The model under review builds one solid part; all positions refer to its coordinate system, in mm. Face numbers are marked on the shaded views. A direction names the side the tool comes from. Coordinates: 2 decimals unless noted, no trailing zeros. Write each loop counter-clockwise with the first axis right and the second up, starting at its lowest first coordinate (ties: lowest second). Pieces come first, ordered by that corner, then holes. Notation, with made-up numbers: (11, -31) - (22, -31) arc R18 ccw to (22, -13) - close; hole circle Ø10 at (62, 86.5). An arc over 180 degrees is marked (long way). Return JSON: item names as keys, results as strings. Group by question number.
(1) We need section B-B on z = 4.25. State the section outline as (x, y) points.
(2) Draft analysis for pull direction Y (two halves, no side actions). For the marked faces 1, 2 and 3, state which applies: released by +Y, released by -Y, zero draft, split by the parting line, or undercut.
(3) Tool access review of the marked faces 4, 5, 6 and 7: name each direction out of +Z, -Z, +X, -X, +Y, -Y from which nothing blocks a thin tool from reaching the whole face with its end or side.
(4) For pin 1 Ø6.5 at (x, y) = (-31, -5) entering from +Z; pin 2 Ø4 at (x, y) = (-38.5, -3) entering from -Z; pin 3 Ø2 at (x, y) = (-10.5, 3.5) entering from +Z, all flat-tipped, find the tip position at first contact; note any pin that passes through.
(5) We need section A-A on x = 0. State the section outline as (y, z) points, then the cut area to 4 significant figures.
(6) We need section C-C on y = -14.75. State the section outline as (x, z) points, then the cut area to 3 significant figures.
(7) To check wall thickness, follow L1, parallel to Y at x = -14, z = 0.75; L2, parallel to Y at x = 2.5, z = 7.5; L3, parallel to Z at x = -11.5, y = 6.5. State the ranges of each line that lie inside material, in increasing order. Write a range as from..to.
(8) We need section D-D on x = -22.5. State the section outline as (y, z) points, then the cut area to 3 significant figures.
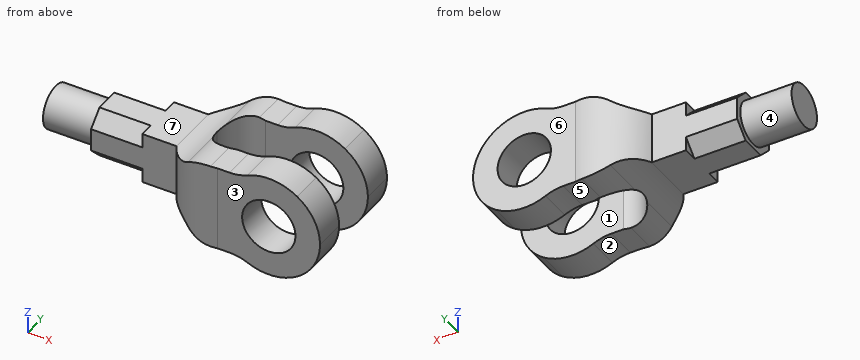
```python
from build123d import *

# Parameters (mm, degrees)
SKETCH4_R               = 12
SKETCH4_R_2             = 6.25
BOSS_EXTRUDE2_DEPTH     = 7.5
BOSS_EXTRUDE3_DEPTH     = 10
SKETCH6_R               = 6.25
CUT_EXTRUDE1_DEPTH      = 20
SKETCH7_W               = 20
SKETCH7_H               = 7.5
BOSS_EXTRUDE4_DEPTH     = 5.36675
CUT_EXTRUDE2_DEPTH      = 50.133277179
CUT_EXTRUDE2_DEPTH_BACK = 50.133277179
FILLET1_R               = 10
FILLET2_R               = 10
CUT_EXTRUDE3_DEPTH      = 12
SKETCH10_R              = 5
BOSS_EXTRUDE5_DEPTH     = 12
FILLET3_R               = 10


with BuildPart() as part:
    # Sketch4 → Boss-Extrude2 (new body)
    with BuildSketch(Plane(origin=(0, 0, 0), x_dir=(1, 0, 0), z_dir=(0, 1, 0))):
        with Locations(Location((0, 0, 0), (0, 0, 270))):
            Circle(SKETCH4_R)
        with Locations(Location((0, 0, 0), (0, 0, 270))):
            Circle(SKETCH4_R_2, mode=Mode.SUBTRACT)
    extrude(amount=BOSS_EXTRUDE2_DEPTH)

    # Sketch5 → Boss-Extrude3 (add, symmetric)
    with BuildSketch(Plane.XY):
        with BuildLine():
            Line((-25.749055866, 0.593145751), (-45.749055866, 0.593145751))
            Line((-45.749055866, 0.593145751), (-45.749055866, -5.656854249))
            Line((-45.749055866, -5.656854249), (-20, -5.656854249))
            ThreePointArc((-20, -5.656854249), (-17.464101615, -0.757874764), (-12, 0))
            Line((-12, 0), (12, 0))
            Line((12, 0), (12, 7.5))
            Line((12, 7.5), (-12, 7.5))
            ThreePointArc((-12, 7.5), (-19.973874913, 6.234976235), (-25.749055866, 0.593145751))
        make_face()
    extrude(amount=BOSS_EXTRUDE3_DEPTH, both=True)

    # Sketch6 → Cut-Extrude1 (cut)
    with BuildSketch(Plane.XZ):
        with BuildLine():
            Line((6.633249581, -10), (12, -10))
            Line((12, -10), (12, 0))
            ThreePointArc((12, 0), (10.573528147, -5.674548662), (6.633249581, -10))
        make_face()
        with BuildLine():
            ThreePointArc((6.633249581, 10), (10.573528147, 5.674548662), (12, 0))
            Line((12, 0), (12, 10))
            Line((12, 10), (6.633249581, 10))
        make_face()
        with BuildLine():
            Line((-12, -10), (-6.633249581, -10))
            ThreePointArc((-6.633249581, -10), (-10.573528147, -5.674548662), (-12, 0))
            Line((-12, 0), (-12, -10))
        make_face()
        with BuildLine():
            ThreePointArc((-12, 0), (-10.573528147, 5.674548662), (-6.633249581, 10))
            Line((-6.633249581, 10), (-12, 10))
            Line((-12, 10), (-12, 0))
        make_face()
        with Locations(Location((0, 0, 0), (0, 0, 270))):
            Circle(SKETCH6_R)
    extrude(amount=-CUT_EXTRUDE1_DEPTH, mode=Mode.SUBTRACT)


with BuildPart() as cut_extrude1_piece_1:
    # of the separate pieces the step leaves, piece 1, a body of its own (cut_extrude1_pieces)
    add(part.part.solids().sort_by_distance((-45.749055866, -5.656854249, 10))[0])



with BuildPart() as cut_extrude1_piece_2:
    # of the separate pieces the step leaves, piece 2, a body of its own (cut_extrude1_pieces)
    add(part.part.solids().sort_by_distance((-6.633249581, 0, 10))[0])


with BuildPart() as cut_extrude1_piece_1_1:
    add(cut_extrude1_piece_1.part)

    add(cut_extrude1_piece_2.part)  # Boss-Extrude4 merges Cut-Extrude1 piece 2
    # Sketch7 → Boss-Extrude4 (add)
    with BuildSketch(Plane(origin=(-12, 0, 0), x_dir=(0, 0, -1), z_dir=(1, 0, 0))):
        with Locations((0, 3.75)):
            Rectangle(SKETCH7_W, SKETCH7_H)
    extrude(amount=BOSS_EXTRUDE4_DEPTH)

    # Mirror2: Cut-Extrude1 piece 1 across plane


with BuildPart() as cut_extrude1_piece_1_2:
    add(cut_extrude1_piece_1_1.part)
    add(cut_extrude1_piece_1_1.part.mirror(Plane(origin=(-45.749055866, -5.656854249, 10), x_dir=(0, 0, 1), z_dir=(0, 1, 0))))

    # Sketch8 → Cut-Extrude2 (cut, two sides: drawn at the far end of the back side and taken through both)
    with BuildSketch(Plane(origin=(0, -5.656854249, 0), x_dir=(-1, 0, 0), z_dir=(0, -1, 0)).offset(-CUT_EXTRUDE2_DEPTH_BACK)):
        with BuildLine():
            ThreePointArc((17.507339718, 10), (21.168502268, 7.052829994), (25.749055866, 6))
            Line((25.749055866, 6), (45.749055866, 6))
            Line((45.749055866, 6), (45.749055866, 10))
            Line((45.749055866, 10), (17.507339718, 10))
        make_face()
        with BuildLine():
            Line((45.749055866, -10), (45.749055866, -6))
            Line((45.749055866, -6), (25.749055866, -6))
            ThreePointArc((25.749055866, -6), (21.168502268, -7.052829994), (17.507339718, -10))
            Line((17.507339718, -10), (45.749055866, -10))
        make_face()
    extrude(amount=CUT_EXTRUDE2_DEPTH + CUT_EXTRUDE2_DEPTH_BACK, mode=Mode.SUBTRACT)

    # Fillet1
    # the kernel refuses this fillet: 10 mm, written as the material it takes off along each edge
    with BuildSketch(Plane(origin=(-17.507339718, -28.296259364, -10), x_dir=(1, 0, 0), z_dir=(0, 1, 0)), Plane(origin=(-17.507339718, -10.590642804, -10), x_dir=(1, 0, 0), z_dir=(0, 1, 0))) as fillet1_piece_1:
        with BuildLine():
            CenterArc((3.920762426, -10), FILLET1_R, 90, 36.410037128)
            ThreePointArc((-2.014836369, -1.952101707), (-0.941870787, -1.043704746), (0, 0))
            Line((0, 0), (3.920762426, 0))
        make_face()
    extrude(amount=27.573193669, mode=Mode.SUBTRACT)

    # Fillet2
    # the kernel refuses this fillet: 10 mm, written as the material it takes off along each edge
    with BuildSketch(Plane(origin=(-17.507339718, -10.590642804, 10), x_dir=(-0.718199432618455, 0, -0.6958373193401812), z_dir=(0, 1, 0))) as fillet2_piece_1:
        with BuildLine():
            CenterArc((4.142483844, -9.910207143), FILLET2_R, 97.683941218, 36.410037128)
            Line((-2.81588935, -2.728212816), (0, 0))
            ThreePointArc((0, 0), (1.402699778, -0.094199313), (2.805399556, 0))
        make_face()
    extrude(amount=27.573193669, mode=Mode.SUBTRACT)
    with BuildSketch(Plane(origin=(-17.507339718, -28.296259364, 10), x_dir=(1, 0, 0), z_dir=(0, 1, 0))) as fillet2_piece_2:
        with BuildLine():
            CenterArc((3.920762426, 10), FILLET2_R, 233.589962872, 36.410037128)
            ThreePointArc((-2.014836369, 1.952101707), (-0.941870787, 1.043704746), (0, 0))
            Line((0, 0), (3.920762426, 0))
        make_face()
    extrude(amount=27.573193669, mode=Mode.SUBTRACT)

    # Sketch9 → Cut-Extrude3 (cut)
    with BuildSketch(Plane.ZY.offset(45.749055866)):
        Polygon((-6, -2.740187583), (-2.666666667, 0.593145751), (-6, 0.593145751), align=None)
        Polygon((6, 0.593145751), (2.666666667, 0.593145751), (6, -2.740187583), align=None)
        Polygon((6, -8.573520916), (6, -11.906854249), (2.666666667, -11.906854249), align=None)
        Polygon((-6, -8.573520916), (-6, -11.906854249), (-2.666666667, -11.906854249), align=None)
    extrude(amount=-CUT_EXTRUDE3_DEPTH, mode=Mode.SUBTRACT)

    # Sketch10 → Boss-Extrude5 (add)
    with BuildSketch(Plane.ZY.offset(45.749055866)):
        with Locations((0, -5.656854249)):
            Circle(SKETCH10_R)
    extrude(amount=BOSS_EXTRUDE5_DEPTH)

    # Fillet3
    fillet3_edges = [cut_extrude1_piece_1_2.edges().sort_by_distance(p)[0] for p in [
        (-6.633249581, 3.75, 10),
        (-6.633249581, 3.75, -10),
        (-6.633249581, -15.063708499, -10),
        (-6.633249581, -15.063708499, 10),
    ]]
    fillet(fillet3_edges, radius=FILLET3_R)


solid = cut_extrude1_piece_1_2.part
```
Ans:
{
 "1": {"outline": "(-57.75, -8.29) - (-45.75, -8.29) - (-45.75, -10.32) - (-33.75, -10.32) - (-33.75, -11.91) - (-25.75, -11.91) arc R13.31 ccw to (-12, -18.81) - (-4.58, -18.81) - (-4.58, -11.31) - (-12, -11.31) arc R6 cw (long way) to (-12, 0) - (-4.58, 0) - (-4.58, 7.5) - (-12, 7.5) arc R13.31 ccw to (-25.75, 0.59) - (-33.75, 0.59) - (-33.75, -0.99) - (-45.75, -0.99) - (-45.75, -3.02) - (-57.75, -3.02) - close; (4.58, -18.81) - (11.22, -18.81) - (11.22, -11.31) - (4.58, -11.31) - close; (4.58, 0) - (11.22, 0) - (11.22, 7.5) - (4.58, 7.5) - close"},
 "2": {"face 1": "undercut", "face 2": "zero draft", "face 3": "released by -Y"},
 "3": {"face 4": "-X", "face 5": "-Z, -X, +Y, -Y", "face 6": "+Z, -Z, +X, +Y", "face 7": "+Z, -X, +Y, -Y"},
 "4": {"pin 1": "z = 6", "pin 2": "z = -6", "pin 3": "z = 10"},
 "5": {"outline": "(-18.81, -12) - (-11.31, -12) - (-11.31, -6.25) - (-18.81, -6.25) - close; (-18.81, 6.25) - (-11.31, 6.25) - (-11.31, 12) - (-18.81, 12) - close; (0, -12) - (7.5, -12) - (7.5, -6.25) - (0, -6.25) - close; (0, 6.25) - (7.5, 6.25) - (7.5, 12) - (0, 12) - close", "area": "172.5 mm²"},
 "6": {"outline": "(-23.72, -6.2) arc R10.49 cw to (-19.52, -8.05) arc R10 ccw to (-13.59, -10) - (-9.17, -10) arc R10 cw to (-5, -10.91) arc R12 ccw (long way) to (-5, 10.91) arc R10 cw to (-9.17, 10) - (-13.59, 10) arc R10 ccw to (-19.52, 8.05) arc R10.49 cw to (-23.72, 6.2) - close; hole circle Ø12.5 at (0, 0)", "area": "564 mm²"},
 "7": {"L1": "-18.96..-11.66, 0.34..7.65", "L2": "-18.81..-11.31, 0..7.5", "L3": "-10..10"},
 "8": {"outline": "(-15.9, -6.52) - (4.58, -6.52) - (4.58, 6.52) - (-15.9, 6.52) - close", "area": "267 mm²"}
}
